Here's how the part is built. I have some questions about the finished solid (model axes, mm). Face numbers are marked on the shaded views. Round coordinates to 2 decimals unless told otherwise and drop trailing zeros. Write each loop counter-clockwise with the first axis right and the second up, starting at its lowest first coordinate (ties: lowest second). Pieces come first, ordered by that corner, then holes. Notation, with made-up numbers: (-17.75, 76) -> (9.25, 76) arc R19 cw to (9.25, 83) -> close; hole circle Ø5 at (-24.75, 12.25). An arc over 180 degrees is marked (long way). Answer as CSV lines item,"result".
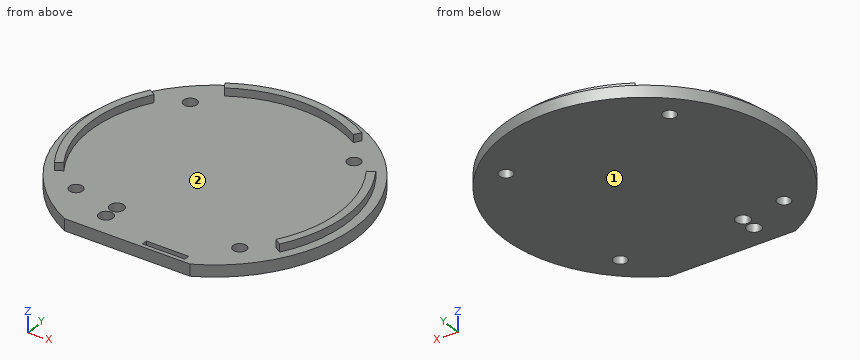
```python
from build123d import *

# Parameters (mm, degrees)
BOSS_EXTRUDE1_DEPTH = 3
SKETCH2_R           = 1.7
CUT_EXTRUDE1_DEPTH  = 3
BOSS_EXTRUDE2_DEPTH = 2
SKETCH6_R           = 1.8
CUT_EXTRUDE2_DEPTH  = 3
SKETCH8_W           = 10.85
SKETCH8_H           = 1.4
CUT_EXTRUDE4_DEPTH  = 1.3


with BuildPart() as part:
    # Sketch1 → Boss-Extrude1 (new body)
    with BuildSketch(Plane.XY):
        with BuildLine():
            Line((-16.06, -32.453666973), (16.06, -32.453666973))
            ThreePointArc((16.06, -32.453666973), (0, 36.21), (-16.06, -32.453666973))
        make_face()
    extrude(amount=BOSS_EXTRUDE1_DEPTH)

    # Sketch2 → Cut-Extrude1 (cut)
    with BuildSketch(Plane.XY.offset(3)):
        with Locations((-20.955, 21.12)):
            Circle(SKETCH2_R)
        with Locations((20.955, 21.12)):
            Circle(SKETCH2_R)
        with Locations((-20.955, -21.12)):
            Circle(SKETCH2_R)
        with Locations((20.955, -21.12)):
            Circle(SKETCH2_R)
    extrude(amount=-CUT_EXTRUDE1_DEPTH, mode=Mode.SUBTRACT)

    # Sketch4 → Boss-Extrude2 (add)
    with BuildSketch(Plane.XY.offset(3)):
        with BuildLine():
            Line((-17.534144761, 28.989794195), (-16.499071281, 27.278472224))
            ThreePointArc((-16.499071281, 27.278472224), (0, 31.88), (16.499071281, 27.278472224))
            Line((16.499071281, 27.278472224), (17.534144761, 28.989794195))
            ThreePointArc((17.534144761, 28.989794195), (0, 33.88), (-17.534144761, 28.989794195))
        make_face()
        with BuildLine():
            Line((-28.851381969, 17.760972903), (-27.148230731, 16.712509332))
            ThreePointArc((-27.148230731, 16.712509332), (-31.88, 0), (-27.148230731, -16.712509332))
            Line((-27.148230731, -16.712509332), (-28.851381969, -17.760972903))
            ThreePointArc((-28.851381969, -17.760972903), (-33.88, 0), (-28.851381969, 17.760972903))
        make_face()
        with BuildLine():
            Line((28.851381969, 17.760972903), (27.148230731, 16.712509332))
            ThreePointArc((27.148230731, 16.712509332), (31.88, 0), (27.148230731, -16.712509332))
            Line((27.148230731, -16.712509332), (28.851381969, -17.760972903))
            ThreePointArc((28.851381969, -17.760972903), (33.88, 0), (28.851381969, 17.760972903))
        make_face()
    extrude(amount=BOSS_EXTRUDE2_DEPTH)

    # Sketch6 → Cut-Extrude2 (cut)
    with BuildSketch(Plane(origin=(0, 0, 0), x_dir=(-1, 0, 0), z_dir=(0, 0, -1))):
        with Locations((9.56, -22.453666973)):
            Circle(SKETCH6_R)
        with Locations((9.56, -26.523666973)):
            Circle(SKETCH6_R)
    extrude(amount=-CUT_EXTRUDE2_DEPTH, mode=Mode.SUBTRACT)

    # Sketch8 → Cut-Extrude4 (cut)
    with BuildSketch(Plane.XY.offset(3)):
        with Locations((8.635, -30.753666973)):
            Rectangle(SKETCH8_W, SKETCH8_H)
    extrude(amount=-CUT_EXTRUDE4_DEPTH, mode=Mode.SUBTRACT)


solid = part.part
```
1. Suppose I cut it at D-D on x = -9.56. Please give me the cut outline in (y, z).
Numbers:
outline,"(-32.45, 0) -> (-28.32, 0) -> (-28.32, 3) -> (-32.45, 3) -> close; (-24.72, 0) -> (-24.25, 0) -> (-24.25, 3) -> (-24.72, 3) -> close; (-20.65, 0) -> (34.93, 0) -> (34.93, 3) -> (32.5, 3) -> (32.5, 5) -> (30.41, 5) -> (30.41, 3) -> (-20.65, 3) -> close"
2. If we mould it in two halves opening along X, with no side actions, what happens to the marked faces 1 and 2? For each: released by +X, released by -X, zero draft, split by the parting line, or undercut.
Numbers:
face 1,"zero draft"
face 2,"undercut"
3. If I drill on line 1 (Y direction, x = -9.56, z = 1.05); line 2 (X direction, y = -21, z = 0.35); line 3 (Z direction, x = 15.5, y = -5), over which ranges is the centre line in solid material (lowest first)?
Numbers:
line 1,"y = -32.45 to -28.32, -24.72 to -24.25, -20.65 to 34.93"
line 2,"x = -29.5 to -22.65, -19.26 to -10.62, -8.5 to 19.26, 22.65 to 29.5"
line 3,"z = 0 to 3"
4. Suppose I cut it at C-C on y = 21.12. Please give me the cut outline in (x, z) (3 decimals), and give its area (3 significant figures).
Numbers:
outline,"(-29.413, 0) -> (-22.655, 0) -> (-22.655, 3) -> (-29.413, 3) -> close; (-19.255, 0) -> (19.255, 0) -> (19.255, 3) -> (-19.255, 3) -> close; (22.655, 0) -> (29.413, 0) -> (29.413, 3) -> (22.655, 3) -> close"
area,"156 mm^2"
5. Suppose I cut it at B-B on x = 0. Please give me the cut outline in (y, z).
Numbers:
outline,"(-32.45, 0) -> (36.21, 0) -> (36.21, 3) -> (33.88, 3) -> (33.88, 5) -> (31.88, 5) -> (31.88, 3) -> (-32.45, 3) -> close"
6. Suppose I cut it at A-A on z = 4.05. Please give me the cut outline in (x, y).
Numbers:
outline,"(-28.85, -17.76) -> (-27.15, -16.71) arc R31.88 cw to (-27.15, 16.71) -> (-28.85, 17.76) arc R33.88 ccw to start; (-17.53, 28.99) -> (-16.5, 27.28) arc R31.88 cw to (16.5, 27.28) -> (17.53, 28.99) arc R33.88 ccw to start; (27.15, -16.71) -> (28.85, -17.76) arc R33.88 ccw to (28.85, 17.76) -> (27.15, 16.71) arc R31.88 cw to start"
7. For pin 1 Ø6 at (x, y) = (-9.56, -26.52) entering from +Z; pin 2 Ø1.4 at (y, z) = (-31, 2.5) entering from -X; pin 3 Ø1.4 at (y, z) = (-31, 2.5) entering from +X, each with a flat end and sliding along its axis, tell me the tip position at first contact or that it passes through.
Numbers:
pin 1,"stops at z = 3"
pin 2,"stops at x = -19.83"
pin 3,"stops at x = 19.83"
